from build123d import *

# Parameters (mm, degrees)
SKETCH1_W           = 6
SKETCH1_H           = 35
BOSS_EXTRUDE1_DEPTH = 20
SKETCH2_W           = 35
SKETCH2_H           = 7
BOSS_EXTRUDE2_DEPTH = 9
SKETCH6_R           = 2.15
CUT_EXTRUDE1_DEPTH  = 16
SKETCH7_W           = 6
SKETCH7_H           = 8
BOSS_EXTRUDE3_DEPTH = 8
SKETCH8_R           = 2.15
CUT_EXTRUDE2_DEPTH  = 16
SKETCH9_W           = 9
SKETCH9_H           = 10
BOSS_EXTRUDE4_DEPTH = 12
CUT_EXTRUDE3_REACH  = 17
SKETCH10_W          = 5
SKETCH10_H          = 40
SKETCH11_W          = 30
SKETCH11_H          = 21
CUT_EXTRUDE4_DEPTH  = 0.7
SKETCH12_W          = 8
SKETCH12_H          = 8
CUT_EXTRUDE5_DEPTH  = 0.7


with BuildPart() as part:
    # Sketch1 → Boss-Extrude1 (new body, symmetric)
    with BuildSketch(Plane(origin=(0, 0, 0), x_dir=(1, 0, 0), z_dir=(0, 1, 0))):
        with Locations((-9.580645161, 13.951612903)):
            Rectangle(SKETCH1_W, SKETCH1_H)
    extrude(amount=BOSS_EXTRUDE1_DEPTH, both=True)

    # Sketch2 → Boss-Extrude2 (add)
    with BuildSketch(Plane(origin=(-6.580645161, 0, 0), x_dir=(0, 0, -1), z_dir=(1, 0, 0))):
        with Locations((13.951612903, 16.5)):
            Rectangle(SKETCH2_W, SKETCH2_H)
    extrude(amount=BOSS_EXTRUDE2_DEPTH)

    # Sketch6 → Cut-Extrude1 (cut, through all)
    with BuildSketch(Plane(origin=(2.419354839, 0, 0), x_dir=(0, 0, -1), z_dir=(1, 0, 0))):
        with Locations((13.451612903, 16.5)):
            Circle(SKETCH6_R)
    extrude(amount=-CUT_EXTRUDE1_DEPTH, mode=Mode.SUBTRACT)

    # Sketch7 → Boss-Extrude3 (add)
    with BuildSketch(Plane(origin=(0, 0, -31.451612903), x_dir=(-1, 0, 0), z_dir=(0, 0, -1))):
        with Locations((9.580645161, -16)):
            Rectangle(SKETCH7_W, SKETCH7_H)
    extrude(amount=BOSS_EXTRUDE3_DEPTH)

    # Sketch8 → Cut-Extrude2 (cut, through all)
    with BuildSketch(Plane.ZY.offset(12.580645161)):
        with Locations((-35.451612903, -16)):
            Circle(SKETCH8_R)
    extrude(amount=-CUT_EXTRUDE2_DEPTH, mode=Mode.SUBTRACT)

    # Sketch9 → Boss-Extrude4 (add)
    with BuildSketch(Plane.XZ.offset(-13)):
        with Locations((-2.080645161, -26.451612903)):
            Rectangle(SKETCH9_W, SKETCH9_H)
    extrude(amount=BOSS_EXTRUDE4_DEPTH)

    # Sketch10 → Cut-Extrude3 (cut, up to next)
    with BuildSketch(Plane.ZY.offset(12.580645161), mode=Mode.PRIVATE) as cut_extrude3_sk1:
        with Locations((1.048387097, 0)):
            Rectangle(SKETCH10_W, SKETCH10_H)
    cut_extrude3_tool1 = extrude(cut_extrude3_sk1.sketch, amount=-CUT_EXTRUDE3_REACH, mode=Mode.PRIVATE) & part.part
    add(cut_extrude3_tool1.solids().sort_by_distance((-12.580645, 0, 1.048387))[0], mode=Mode.SUBTRACT)

    # Sketch11 → Cut-Extrude4 (cut)
    with BuildSketch(Plane(origin=(-6.580645161, 0, 0), x_dir=(0, 0, -1), z_dir=(1, 0, 0))):
        with Locations((16.451612903, -9.5)):
            Rectangle(SKETCH11_W, SKETCH11_H)
    extrude(amount=-CUT_EXTRUDE4_DEPTH, mode=Mode.SUBTRACT)

    # Sketch12 → Cut-Extrude5 (cut)
    with BuildSketch(Plane(origin=(-6.580645161, 0, 0), x_dir=(0, 0, -1), z_dir=(1, 0, 0))):
        with Locations((35.451612903, -16)):
            Rectangle(SKETCH12_W, SKETCH12_H)
    extrude(amount=-CUT_EXTRUDE5_DEPTH, mode=Mode.SUBTRACT)


solid = part.part
Read the model definition and answer for the solid it produces. Units are mm, in the model's axes. A direction names the side the tool comes from. Give positions to 0.01 mm unless a question says otherwise; leave off trailing zeros. Write each loop counter-clockwise with the first axis right and the second up, starting at its lowest first coordinate (ties: lowest second). Pieces come first, ordered by that corner, then holes. Notation, with made-up numbers: (18, -27.75) -> (67, -27.75) arc R19 ccw to (67, -21.75) -> close; hole circle Ø9 at (36.5, -12). An arc over 180 degrees is marked (long way). Answer as a JSON object with one key per item and string values. Group by question number.
1) A tool of negligible diameter and unlimited length cuts with its end or side. For faces 4 (the flat face through (-12.581, 0, -16)), 5 (the flat face through (-7, 8, -31.452)), 6 (the flat face through (-4, 1, -23)), 7 (the flat face through (-6.581, 7, -11)), from which of +Z, -Z, +X, -X, +Y, -Y can it reach the whole face along a straight path? Write none if from no direction.
2) The mould has two halves that part along Z. Classify faces 1 (the flat face through (-10, -12, -35)), 2 (the flat face through (-2, 7, -21.452)), 3 (the cylindrical face through (-9.968, -17.907, -34.46)): +Z half, -Z half, draft (parallel to the pull), parting line (faces both ways), or undercut.
3) Find section A-A (y = 16.5). Write down the section's boundary in (x, z).
4) Each of these flat-tipped pins is pushed along its axis until it touches: P1, Ø4.5, axis at x = -5.5, y = 1.5, coming from the -Z side; P2, Ø1, axis at y = 10.5, z = -9, coming from the +X side; P3, Ø10.5, axis at y = -12.5, z = -12.5, coming from the +X side; P4, Ø3, axis at x = -2, z = -34, coming from the -Y side. Where does it stop, or does it pass through?
5) Find section C-C (z = -27.5). Write down the section's boundary in (x, y), and give its area (3 significant figures).
6) Find section B-B (x = 1.5). Write down the section's boundary in (y, z), and give its area (3 significant figures).
7) Consider L1, parallel to X at y = -6, z = -13; L2, parallel to Y at x = -7.75, z = -31.5; L3, parallel to Y at x = 0.5, z = -13.5. Determine where each line is inside the solid, lowest interval first. Write a range as from..to.
8) Find section D-D (y = -16). Write down the section's boundary in (x, z).
Values follow:
{
 "1": {"face 4": "+Z, -Z, -X, +Y, -Y", "face 5": "-Z, +X, -X, +Y", "face 6": "+Z, -Z, +X, -Y", "face 7": "+Z, +X, -Y"},
 "2": {"face 1": "draft", "face 2": "+Z half", "face 3": "undercut"},
 "3": {"outline": "(-12.58, -31.45) -> (2.42, -31.45) -> (2.42, -15.6) -> (-12.58, -15.6) -> close; (-12.58, -11.3) -> (2.42, -11.3) -> (2.42, -1.45) -> (-12.58, -1.45) -> close"},
 "4": {"P1": "stops at z = -31.45", "P2": "stops at x = -6.58", "P3": "stops at x = -7.28", "P4": "passes through"},
 "5": {"outline": "(-12.58, -20) -> (-7.28, -20) -> (-7.28, 1) -> (2.42, 1) -> (2.42, 20) -> (-12.58, 20) -> close", "area": "396 mm2"},
 "6": {"outline": "(1, -31.45) -> (20, -31.45) -> (20, -1.45) -> (13, -1.45) -> (13, -21.45) -> (1, -21.45) -> close; hole circle Ø4.3 at (16.5, -13.45)", "area": "315 mm2"},
 "7": {"L1": "x = -12.58..-7.28", "L2": "y = -20..-12", "L3": "y = 13..14.35, 18.65..20"},
 "8": {"outline": "(-12.58, -39.45) -> (-7.28, -39.45) -> (-7.28, -37.6) -> (-12.58, -37.6) -> close; (-12.58, -33.3) -> (-7.28, -33.3) -> (-7.28, -1.45) -> (-12.58, -1.45) -> close"}
}
